CAD build for the part. Positions are in the model's coordinates, mm. Face numbers are marked on the shaded views. A direction names the side the tool comes from. Coordinates: 2 decimals unless noted, no trailing zeros. Loops run counter-clockwise (first coordinate to the right, second up) from the corner with the lowest first, then second, coordinate; pieces in that order, holes last. Notation, with made-up numbers: (58, -32) -> (67, -32) arc R16 ccw to (67, -8) -> close; hole circle Ø10 at (-0.75, 22.25). An arc over 180 degrees is marked (long way). Answer as a JSON object with one key per item and string values. Group by question number.
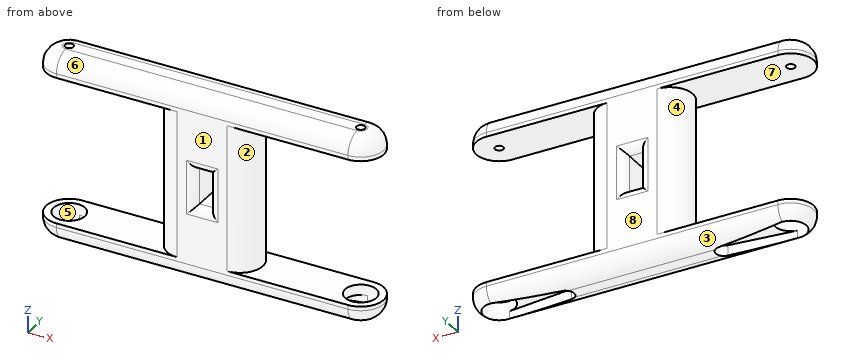
from build123d import *

# Parameters (mm, degrees)
BOSS_EXTRU_1_DEPTH      = 1
BOSS_EXTRU_1_DEPTH_BACK = 4
ESQUISSE1_R             = 3.75
ENL_V_MAT_EXTRU_1_DEPTH = 2.5
BOSS_EXTRU_2_DEPTH      = 35.2
BOSS_EXTRU_3_START      = 5
BOSS_EXTRU_3_DEPTH      = 5
ESQUISSE5_R             = 1
ENL_V_MAT_EXTRU_2_DEPTH = 5
CONG_1_R                = 4
ESQUISSE6_W             = 3.5
ESQUISSE6_H             = 9
ENL_V_MAT_EXTRU_3_DEPTH = 2089.490019804
CONG_2_R                = 2


with BuildPart() as part:
    # Esquisse1 → Boss.-Extru.1 (new, two sides: drawn at the far end of the back side and taken through both)
    with BuildSketch(Plane(origin=(0, 0, 2042.895904074), x_dir=(-1, 0, 0), z_dir=(0, 0, -1)).offset(-BOSS_EXTRU_1_DEPTH_BACK)):
        with BuildLine():
            Line((0, -5.5), (-70, -5.5))
            ThreePointArc((-70, -5.5), (-75.5, 0), (-70, 5.5))
            Line((-70, 5.5), (0, 5.5))
            ThreePointArc((0, 5.5), (5.5, 0), (0, -5.5))
        make_face()
        Circle(ESQUISSE1_R, mode=Mode.SUBTRACT)
        with Locations((-70, 0)):
            Circle(ESQUISSE1_R, mode=Mode.SUBTRACT)
    extrude(amount=BOSS_EXTRU_1_DEPTH + BOSS_EXTRU_1_DEPTH_BACK)

    # Esquisse2 → Enlèv. mat.-Extru.1 (cut)
    with BuildSketch(Plane(origin=(0, 0, 2041.895904074), x_dir=(-1, 0, 0), z_dir=(0, 0, -1))):
        with BuildLine():
            Line((-0.41015625, -3.727502093), (-16.21875, -1.988001116))
            ThreePointArc((-16.21875, -1.988001116), (-18, 0), (-16.21875, 1.988001116))
            Line((-16.21875, 1.988001116), (-0.41015625, 3.727502093))
            Line((-0.41015625, 3.727502093), (-0.41015625, -3.727502093))
        make_face()
        with BuildLine():
            Line((-53.78125, 1.988001116), (-69.58984375, 3.727502093))
            Line((-69.58984375, 3.727502093), (-69.58984375, -3.727502093))
            Line((-69.58984375, -3.727502093), (-53.78125, -1.988001116))
            ThreePointArc((-53.78125, -1.988001116), (-52, 0), (-53.78125, 1.988001116))
        make_face()
    extrude(amount=-ENL_V_MAT_EXTRU_1_DEPTH, mode=Mode.SUBTRACT)

    # Esquisse3 → Boss.-Extru.2 (add)
    with BuildSketch(Plane.XY.offset(2046.895904074)):
        with BuildLine():
            Line((29, 5.5), (41, 5.5))
            ThreePointArc((41, 5.5), (46.5, 0), (41, -5.5))
            Line((41, -5.5), (29, -5.5))
            ThreePointArc((29, -5.5), (23.5, 0), (29, 5.5))
        make_face()
    extrude(amount=BOSS_EXTRU_2_DEPTH)

    # Esquisse4 → Boss.-Extru.3 (add)
    with BuildSketch(Plane.XY.offset(2082.095904074).offset(BOSS_EXTRU_3_START)):
        with BuildLine():
            Line((0, 5.5), (70, 5.5))
            ThreePointArc((70, 5.5), (75.5, 0), (70, -5.5))
            Line((70, -5.5), (0, -5.5))
            ThreePointArc((0, -5.5), (-5.5, 0), (0, 5.5))
        make_face()
    extrude(amount=-BOSS_EXTRU_3_DEPTH)

    # Esquisse5 → Enlèv. mat.-Extru.2 (cut)
    with BuildSketch(Plane.XY.offset(2087.095904074)):
        Circle(ESQUISSE5_R)
        with Locations((70, 0)):
            Circle(ESQUISSE5_R)
    extrude(amount=-ENL_V_MAT_EXTRU_2_DEPTH, mode=Mode.SUBTRACT)

    # Congé1
    # the kernel refuses this fillet: 4 mm, written as the material it takes off along each edge
    with BuildSketch(Plane(origin=(70, 5.5, 2041.895904074), x_dir=(0, 0, 1), z_dir=(-1, 0, 0)), Plane(origin=(0, -5.5, 2041.895904074), x_dir=(0, 0, 1), z_dir=(1, 0, 0)), Plane(origin=(70, -5.5, 2087.095904074), x_dir=(0, 0, -1), z_dir=(-1, 0, 0)), Plane(origin=(0, 5.5, 2087.095904074), x_dir=(0, 0, -1), z_dir=(1, 0, 0))) as cong_1_piece_1:
        with BuildLine():
            CenterArc((CONG_1_R, -CONG_1_R), CONG_1_R, 90, 90)
            Line((0, -CONG_1_R), (0, 0))
            Line((0, 0), (CONG_1_R, 0))
        make_face()
    extrude(amount=70, mode=Mode.SUBTRACT)
    with BuildSketch(Plane(origin=(70, 0, 2087.095904074), x_dir=(0, 1, 0), z_dir=(-1, 0, 0))) as cong_1_piece_2:
        with BuildLine():
            CenterArc((5.5 - CONG_1_R, CONG_1_R), CONG_1_R, 270, 90)
            Line((5.5, CONG_1_R), (5.5, 0))
            Line((5.5, 0), (5.5 - CONG_1_R, 0))
        make_face()
    revolve(axis=Axis((70, 0, 2087.095904074), (0, 0, -1)), revolution_arc=180, mode=Mode.SUBTRACT)
    with BuildSketch(Plane(origin=(0, 0, 2087.095904074), x_dir=(0, -1, 0), z_dir=(1, 0, 0))) as cong_1_piece_3:
        with BuildLine():
            CenterArc((5.5 - CONG_1_R, CONG_1_R), CONG_1_R, 270, 90)
            Line((5.5 - CONG_1_R, 0), (5.5, 0))
            Line((5.5, 0), (5.5, CONG_1_R))
        make_face()
    revolve(axis=Axis((0, 0, 2087.095904074), (0, 0, -1)), revolution_arc=180, mode=Mode.SUBTRACT)
    with BuildSketch(Plane(origin=(0, 0, 2041.895904074), x_dir=(0, 1, 0), z_dir=(1, 0, 0))) as cong_1_piece_4:
        with BuildLine():
            CenterArc((5.5 - CONG_1_R, CONG_1_R), CONG_1_R, 270, 90)
            Line((5.5, CONG_1_R), (5.5, 0))
            Line((5.5, 0), (5.5 - CONG_1_R, 0))
        make_face()
    revolve(axis=Axis((0, 0, 2041.895904074), (0, 0, 1)), revolution_arc=180, mode=Mode.SUBTRACT)
    with BuildSketch(Plane(origin=(70, 0, 2041.895904074), x_dir=(0, -1, 0), z_dir=(-1, 0, 0))) as cong_1_piece_5:
        with BuildLine():
            CenterArc((5.5 - CONG_1_R, CONG_1_R), CONG_1_R, 270, 90)
            Line((5.5 - CONG_1_R, 0), (5.5, 0))
            Line((5.5, 0), (5.5, CONG_1_R))
        make_face()
    revolve(axis=Axis((70, 0, 2041.895904074), (0, 0, 1)), revolution_arc=180, mode=Mode.SUBTRACT)

    # Esquisse6 → Enlèv. mat.-Extru.3 (cut, through all)
    with BuildSketch(Plane(origin=(0, 5.5, 0), x_dir=(1, 0, 0), z_dir=(0, 1, 0))):
        with Locations((35, -2064.495904074)):
            Rectangle(ESQUISSE6_W, ESQUISSE6_H)
    extrude(amount=-ENL_V_MAT_EXTRU_3_DEPTH, mode=Mode.SUBTRACT)

    # Congé2
    cong_2_edges = [part.edges().sort_by_distance(p)[0] for p in [
        (36.75, -5.5, 2064.495904074),
        (35, -5.5, 2068.995904074),
        (33.25, -5.5, 2064.495904074),
        (35, -5.5, 2059.995904074),
        (36.75, 5.5, 2064.495904074),
        (35, 5.5, 2059.995904074),
        (33.25, 5.5, 2064.495904074),
        (35, 5.5, 2068.995904074),
    ]]
    fillet(cong_2_edges, radius=CONG_2_R)


solid = part.part
Item 1: Band-saw the part on A-A, the plane x = 48.5. List the corners of the cut face in (y, z), and give its area (3 significant figures).
Item 2: 3-axis set-ups, long thin cutter, end or side, ignore diameter. For the marked faces 1, 2, 3, 4 and 5: which of +Z, -Z, +X, -X, +Y, -Y reach the whole face in a straight line?
Item 3: Band-saw the part on D-D, the plane x = 38. List the corners of the cut face in (y, z).
Item 4: Flat gauge pins, fed straight in: P1, Ø5, axis at y = -4, z = 2070.5, coming from the -X side; P2, Ø1, axis at y = -0.5, z = 2069.5, coming from the +X side; P3, Ø6, axis at x = 0, y = 0, coming from the -Z side. Where does each tip first touch, or does it go through?
Item 5: Band-saw the part on C-C, the plane z = 2051. List the corners of the cut face in (x, y).
Item 6: Pull direction Z, two halves, no side cores. Call the marked faces 6, 7 and 8: +Z half, -Z half, draft (parallel to the pull), parting line (faces both ways), or undercut.
Item 7: Band-saw the part on B-B, the plane x = 60.5. List the corners of the cut face in (y, z).
Item 8: Drill centre lines: L1, parallel to Z at x = 22.5, y = 1.75; L2, parallel to Z at x = 60, y = 1.25; L3, parallel to Y at x = 0, z = 2046. Where is each one in solid material? Low to high.
Reply:
{
 "1": {"outline": "(-5.5, 2045.9) arc R4 ccw to (-1.5, 2041.9) -> (1.5, 2041.9) arc R4 ccw to (5.5, 2045.9) -> (5.5, 2046.9) -> (-5.5, 2046.9) -> close; (-5.5, 2082.1) -> (5.5, 2082.1) -> (5.5, 2083.1) arc R4 ccw to (1.5, 2087.1) -> (-1.5, 2087.1) arc R4 ccw to (-5.5, 2083.1) -> close", "area": "96.3 mm²"},
 "2": {"face 1": "+Z, -Z, +X, -X, -Y", "face 2": "+X", "face 3": "-Z, +X, -X, +Y", "face 4": "-X", "face 5": "-Z"},
 "3": {"outline": "(-5.5, 2045.9) arc R4 ccw to (-1.5, 2041.9) -> (1.5, 2041.9) arc R4 ccw to (5.5, 2045.9) -> (5.5, 2058) arc R2 ccw to (5.35, 2058.75) -> (5.35, 2070.25) arc R2 ccw to (5.5, 2071) -> (5.5, 2083.1) arc R4 ccw to (1.5, 2087.1) -> (-1.5, 2087.1) arc R4 ccw to (-5.5, 2083.1) -> (-5.5, 2071) arc R2 ccw to (-5.35, 2070.25) -> (-5.35, 2058.75) arc R2 ccw to (-5.5, 2058) -> close"},
 "4": {"P1": "x = 23.71", "P2": "x = 46.5", "P3": "z = 2082.1"},
 "5": {"outline": "(29, -5.5) -> (41, -5.5) arc R5.5 ccw to (41, 5.5) -> (29, 5.5) arc R5.5 ccw to start"},
 "6": {"face 6": "+Z half", "face 7": "undercut", "face 8": "draft"},
 "7": {"outline": "(-5.5, 2045.9) arc R4 ccw to (-2.73, 2042.09) -> (-2.73, 2044.4) -> (2.73, 2044.4) -> (2.73, 2042.09) arc R4 ccw to (5.5, 2045.9) -> (5.5, 2046.9) -> (-5.5, 2046.9) -> close; (-5.5, 2082.1) -> (5.5, 2082.1) -> (5.5, 2083.1) arc R4 ccw to (1.5, 2087.1) -> (-1.5, 2087.1) arc R4 ccw to (-5.5, 2083.1) -> close"},
 "8": {"L1": "2041.9 to 2046.9, 2082.1 to 2087.09", "L2": "2044.4 to 2046.9, 2082.1 to 2087.1", "L3": "-5.5 to -3.75, 3.75 to 5.5"}
}
